```python
from build123d import *

# Parameters (mm, degrees)
FILLET1_R = 0.2


with BuildPart() as part:
    # Sketch1 → Revolve1 (revolve)
    with BuildSketch(Plane(origin=(0, 0, 0), x_dir=(0, 0, -1), z_dir=(1, 0, 0))):
        Polygon((0, 0), (-1.75, 0), (-1.75, 9), (2.25, 9), (2.25, 7), (0, 7), align=None)
    revolve(axis=Axis((0, 0, 1.75), (0, 1, 0)))

    # Fillet1
    fillet1_edges = [part.edges().sort_by_distance(p)[0] for p in [
        (0, 7, 5.75),
        (0, 9, 5.75),
        (0, 0, 3.5),
    ]]
    fillet(fillet1_edges, radius=FILLET1_R)


solid = part.part
```
Read the model definition and answer for the solid it produces. Units are mm, in the model's axes. A direction names the side the tool comes from. Coordinates: 2 decimals unless noted, no trailing zeros. Write each loop counter-clockwise with the first axis right and the second up, starting at its lowest first coordinate (ties: lowest second). Pieces come first, ordered by that corner, then holes. Notation, with made-up numbers: (-1, 68.5) -> (7, 68.5) arc R24 cw to (7, 94.5) -> close; hole circle Ø3 at (-28, -19). An arc over 180 degrees is marked (long way). Return JSON: item names as keys, results as strings.
1. Each of these flat-tipped pins is pushed along its axis until it touches: P1, Ø1, axis at x = -1.5, y = 5, coming from the -Z side; P2, Ø1.5, axis at y = 4, z = 1.5, coming from the +X side; P3, Ø1.5, axis at x = 2, y = 6.5, coming from the -Z side. Where does it stop, or does it pass through?
Found:
{"P1": "z = 0.31", "P2": "x = 1.75", "P3": "z = -1.91"}
2. A cutting plane is placed at C-C (y = 4.5). Determine the outline of the cut face in (x, z), and give its area (3 significant figures).
Found:
{"outline": "circle Ø3.5 at (0, 1.75)", "area": "9.62 mm2"}
3. A cutting plane is placed at A-A (x = 0). Determine the outline of the cut face in (y, z).
Found:
{"outline": "(0, 0.2) arc R0.2 ccw to (0.2, 0) -> (7, 0) -> (7, -2.05) arc R0.2 ccw to (7.2, -2.25) -> (8.8, -2.25) arc R0.2 ccw to (9, -2.05) -> (9, 5.55) arc R0.2 ccw to (8.8, 5.75) -> (7.2, 5.75) arc R0.2 ccw to (7, 5.55) -> (7, 3.5) -> (0.2, 3.5) arc R0.2 ccw to (0, 3.3) -> close"}
4. A cutting plane is placed at B-B (z = 1.75). Determine the outline of the cut face in (x, y), and give its area (3 significant figures).
Found:
{"outline": "(-4, 7.2) arc R0.2 ccw to (-3.8, 7) -> (-1.75, 7) -> (-1.75, 0.2) arc R0.2 ccw to (-1.55, 0) -> (1.55, 0) arc R0.2 ccw to (1.75, 0.2) -> (1.75, 7) -> (3.8, 7) arc R0.2 ccw to (4, 7.2) -> (4, 8.8) arc R0.2 ccw to (3.8, 9) -> (-3.8, 9) arc R0.2 ccw to (-4, 8.8) -> close", "area": "40.4 mm2"}
5. Find the intervals of material crossed by line 1 along Y through (x, z) = (2.5, 1.25); line 2 along Z through (x, y) = (0, 5); line 3 along Z through (x, y) = (-1.5, 3.5), in increasing order. Write a range as from..to.
Found:
{"line 1": "7..9", "line 2": "0..3.5", "line 3": "0.85..2.65"}
6. A tool of negligible diameter and unlimited length cuts with its end or side. For faces 1 (the face through (0, 9, 2)), 2 (the face through (-0.526, 3.552, 0.081)), from which of +Z, -Z, +X, -X, +Y, -Y can it reach the whole face along a straight path? Write none if from no direction.
Found:
{"face 1": "+Z, -Z, +X, -X, +Y", "face 2": "-Y"}
